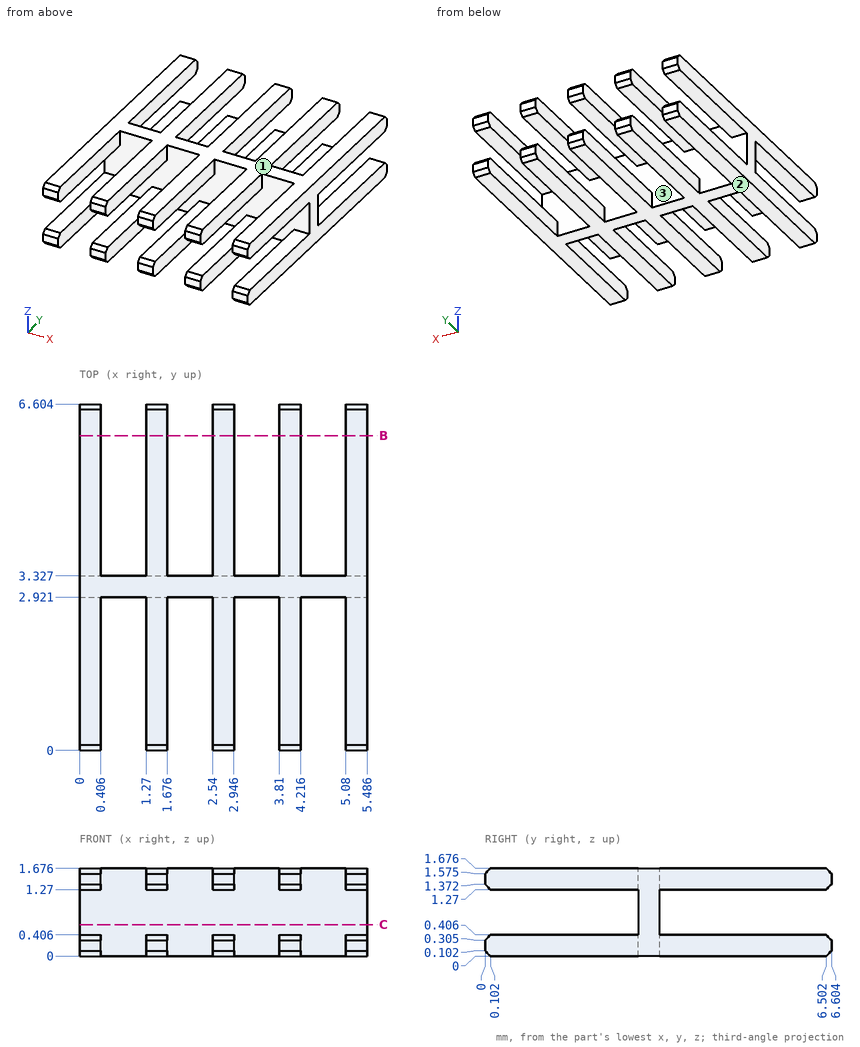
Could you check a few things on this drawing? It's one solid part, dimensions in mm from its lowest x, y, z. Round coordinates to 2 decimals unless told otherwise and drop trailing zeros. Write each loop counter-clockwise with the first axis right and the second up, starting at its lowest first coordinate (ties: lowest second). Pieces come first, ordered by that corner, then holes.
Q1. Please list where these lines run through material, in increasing order: probe 1 along X at (y, z) = (2.25, 1.35); probe 2 along Z at (x, y) = (2.9, 4); probe 3 along Y at (x, z) = (4.5, 0.9).
Q2. If we mould it in two halves opening along Z, with no side actions, what happens to the marked faces 1, 2 and 3? For each: +Z half, -Z half, draft (parallel to the pull), parting line (faces both ways), or undercut.
Q3. If we section it at C-C on z = 0.6: Write out the boundary of the cut face in (x, y).
Q4. If we section it at B-B on y = 6: Give the number of separate pieces and of enclosed holes in the cut face.
Answer below:
1. probe 1: x = 0 to 0.41, 1.27 to 1.68, 2.54 to 2.95, 3.81 to 4.22, 5.08 to 5.49
1. probe 2: z = 0 to 0.41, 1.27 to 1.68
1. probe 3: y = 2.92 to 3.33
2. face 1: +Z half
2. face 2: -Z half
2. face 3: undercut
3. outline: (0, 2.92) - (5.49, 2.92) - (5.49, 3.33) - (0, 3.33) - close
4. separate pieces: 10
4. enclosed holes: 0
